from build123d import *

# Parameters (mm, degrees)
SKETCH1_W            = 30
SKETCH1_H            = 15
BOSS_EXTRUDE1_DEPTH  = 1
M3_CLEARANCE_HOLE1_D = 3.4


with BuildPart() as part:
    # Sketch1 → Boss-Extrude1 (new body)
    with BuildSketch(Plane.XY):
        with Locations((15, 7.5)):
            Rectangle(SKETCH1_W, SKETCH1_H)
    extrude(amount=BOSS_EXTRUDE1_DEPTH)

    # M3 Clearance Hole1 (through all)
    with Locations(Plane(origin=(0, 0, 0), x_dir=(-1, 0, 0), z_dir=(0, 0, -1))):
        with Locations((-15, 7.5)):
            Hole(M3_CLEARANCE_HOLE1_D / 2)


solid = part.part
Can you work these out from the model? Positions are in its coordinate system, mm. Round coordinates to 2 decimals unless told otherwise and drop trailing zeros. Order: outer loops, then holes, each group sorted by start corner. A loop starts at its lowest first (then second) coordinate and runs counter-clockwise, first axis right, second up. Notation, with made-up numbers: (59, 56) -> (95, 56) arc R20 cw to (95, 87) -> close; hole circle Ø7 at (52, 9.5). An arc over 180 degrees is marked (long way). Write each question's results on one line, items separated by ' | '. Start each with the question number.
Item 1: Please list where these lines run through material, in increasing order: L1, parallel to Y at x = 15, z = 0.65; L2, parallel to X at y = 8.25, z = 0.9; L3, parallel to X at y = 7, z = 0.65.
Item 2: Thinking about a two-plate mould opening in Y: for faces 1 (the cylindrical face through (16.57, 6.85, 0.51)), 2 (the flat face through (15, 11, 1)), 3 (the flat face through (14.8, 0, 0.5)), which applies, +Y half, -Y half, draft (parallel to the pull), parting line (faces both ways), or undercut?
Item 3: If we section it at C-C, the plane z = 0.7: Write out the boundary of the cut face in (x, y), then the cut area to 3 significant figures.
Item 4: If we section it at B-B, the plane y = 7.5: Write out the boundary of the cut face in (x, z).
Item 5: If we section it at A-A, the plane x = 15: Write out the boundary of the cut face in (y, z).
Results:
1) L1: y = 0 to 5.8, 9.2 to 15 | L2: x = 0 to 13.47, 16.53 to 30 | L3: x = 0 to 13.38, 16.62 to 30
2) face 1: undercut | face 2: draft | face 3: -Y half
3) outline: (0, 0) -> (30, 0) -> (30, 15) -> (0, 15) -> close; hole circle Ø3.4 at (15, 7.5) | area: 441 mm2
4) outline: (0, 0) -> (13.3, 0) -> (13.3, 1) -> (0, 1) -> close; (16.7, 0) -> (30, 0) -> (30, 1) -> (16.7, 1) -> close
5) outline: (0, 0) -> (5.8, 0) -> (5.8, 1) -> (0, 1) -> close; (9.2, 0) -> (15, 0) -> (15, 1) -> (9.2, 1) -> close
